```python
from build123d import *

# Parameters (mm, degrees)
BOSS_EXTRUDE1_DEPTH = 2
BOSS_EXTRUDE2_START = -0.573063
SKETCH2_R           = 3.25
SKETCH2_R_2         = 1.75
BOSS_EXTRUDE2_DEPTH = 7.073063
BOSS_EXTRUDE3_START = -0.573063
SKETCH3_R           = 3.25
SKETCH3_R_2         = 1.75
BOSS_EXTRUDE3_DEPTH = 7.073063
SKETCH4_R           = 1.5
CUT_EXTRUDE1_DEPTH  = 2
CHAMFER1_SIZE       = 1


with BuildPart() as part:
    # Sketch1 → Boss-Extrude1 (new body)
    with BuildSketch(Plane(origin=(0, 0, 0), x_dir=(1, 0, 0), z_dir=(0, 1, 0))):
        with BuildLine():
            Line((-41.75, 3.25), (41.75, 3.25))
            ThreePointArc((41.75, 3.25), (45, 0), (41.75, -3.25))
            Line((41.75, -3.25), (-41.75, -3.25))
            ThreePointArc((-41.75, -3.25), (-45, 0), (-41.75, 3.25))
        make_face()
    extrude(amount=BOSS_EXTRUDE1_DEPTH)

    # Sketch2 → Boss-Extrude2 (add)
    with BuildSketch(Plane(origin=(-1.600936684, 9.079363113, 0), x_dir=(0, 0, -1), z_dir=(-0.17364817766693072, 0.984807753012208, 0)).offset(BOSS_EXTRUDE2_START)):
        with Locations(Location((0, 40.768427333, 0), (0, 0, 180))):
            Circle(SKETCH2_R)
        with Locations(Location((0, 40.768427333, 0), (0, 0, 270))):
            Circle(SKETCH2_R_2, mode=Mode.SUBTRACT)
    extrude(amount=BOSS_EXTRUDE2_DEPTH)

    # Sketch3 → Boss-Extrude3 (add)
    with BuildSketch(Plane(origin=(1.600936684, 9.079363113, 0), x_dir=(0, 0, -1), z_dir=(0.17364817766693072, 0.984807753012208, 0)).offset(BOSS_EXTRUDE3_START)):
        with Locations((0, -40.768427333)):
            Circle(SKETCH3_R)
        with Locations(Location((0, -40.768427333, 0), (0, 0, 90))):
            Circle(SKETCH3_R_2, mode=Mode.SUBTRACT)
    extrude(amount=BOSS_EXTRUDE3_DEPTH)

    # Sketch4 → Cut-Extrude1 (cut)
    with BuildSketch(Plane(origin=(0, 2, 0), x_dir=(1, 0, 0), z_dir=(0, 1, 0))):
        with Locations(Location((-15, 0, 0), (0, 0, 270))):
            Circle(SKETCH4_R)
        with Locations(Location((15, 0, 0), (0, 0, 270))):
            Circle(SKETCH4_R)
    extrude(amount=-CUT_EXTRUDE1_DEPTH, mode=Mode.SUBTRACT)

    # Chamfer1
    chamfer1_edges = [part.edges().sort_by_distance(p)[0] for p in [
        (-15, 2, -1.5),
        (15, 2, -1.5),
    ]]
    chamfer(chamfer1_edges, length=CHAMFER1_SIZE)


solid = part.part
```
Verification items for the finished model (mm, model axes). A direction names the side the tool comes from. Give positions to 0.01 mm unless a question says otherwise; leave off trailing zeros. Loops run counter-clockwise (first coordinate to the right, second up) from the corner with the lowest first, then second, coordinate; pieces in that order, holes last.
1. Section check C-C, the plane x = -1.5. Enter the section's corners in (y, z).
2. Set-up check for faces 1 (the flat face through (42, 2, 0)), 2 (the cylindrical face through (45, 1, 0)), 3 (the cylindrical face through (-45, 1, 0)): record each of +Z, -Z, +X, -X, +Y, -Y from which the full face is reachable in a straight line by a thin tool's end or side.
3. Mould release check, pull along Z, two halves, no side actions. Record for faces 4 (the flat face through (44.256, 8.158, -1.399)), 5 (the cylindrical face through (39.07, 5.37, 0.42)), 6 (the cylindrical face through (-40.635, 5.292, -0.526)), 7 (the flat face through (-42, 2, 0)): released by +Z, released by -Z, zero draft, split by the parting line, or undercut.
4. Section check B-B, the plane z = 0. Count the separate pieces of the cut face and the enclosed holes in it, then the cut area to 3 significant figures.
5. Go/stop test with flat-tipped pins: pin 1 Ø1.5 at (x, y) = (-35.5, 3) entering from +Z; pin 2 Ø1 at (x, z) = (41.5, 0.5) entering from +Y; pin 3 Ø1.8 at (x, z) = (-42.5, -1) entering from +Y. Record where each tip stops, or that it passes through.
6. Thickness scan on line 1 (X direction, y = 0.2, z = 0); line 2 (X direction, y = 4, z = 0.5); line 3 (X direction, y = 7.25, z = 1.5). Record the ranges inside material, lowest first.
7. Section check A-A, the plane x = 15. Enter the section's corners in (y, z).
Geometry says:
1. outline: (0, -3.25) - (2, -3.25) - (2, 3.25) - (0, 3.25) - close
2. face 1: none
2. face 2: +X, -Y
2. face 3: -X, -Y
3. face 4: zero draft
3. face 5: split by the parting line
3. face 6: undercut
3. face 7: undercut
4. separate pieces: 3
4. enclosed holes: 0
4. area: 205 mm2
5. pin 1: passes through
5. pin 2: stops at y = 8.73
5. pin 3: stops at y = 8.62
6. line 1: x = -45 to -16.5, -13.5 to 13.5, 16.5 to 45
6. line 2: x = -45.36 to -43.81, -40.4 to -38.84, 38.84 to 40.4, 43.81 to 45.36
6. line 3: x = -45.6 to -43.59, -41.76 to -39.75, 39.75 to 41.76, 43.59 to 45.6
7. outline: (0, -3.25) - (2, -3.25) - (2, -2.5) - (1, -1.5) - (0, -1.5) - close; (0, 1.5) - (1, 1.5) - (2, 2.5) - (2, 3.25) - (0, 3.25) - close
